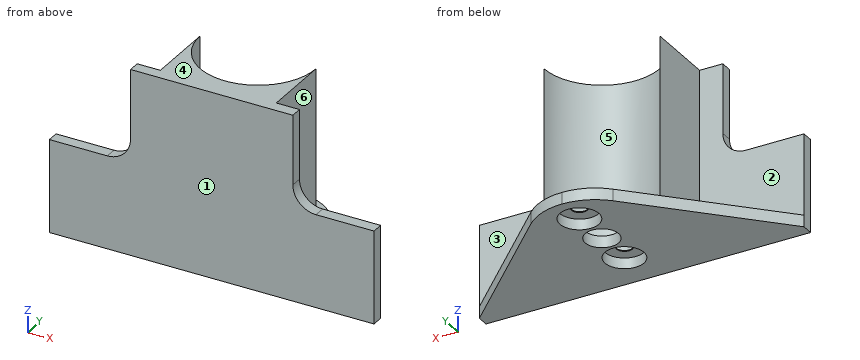
from build123d import *

# Parameters (mm, degrees)
BOSS_EXTRUDE1_DEPTH                              = 2.5
FILLET1_R                                        = 5
SKETCH3_W                                        = 70
SKETCH3_H                                        = 2.5
BOSS_EXTRUDE2_DEPTH                              = 30
CUT_EXTRUDE1_REACH                               = 62.725
BOSS_EXTRUDE3_DEPTH                              = 37.5
CUT_EXTRUDE3_REACH                               = 62.725
SKETCH10_R                                       = 3.6
CBORE_FOR_M3_HEX_HEAD_MACHINE_SCREW1_D           = 3.4
CBORE_FOR_M3_HEX_HEAD_MACHINE_SCREW1_CBORE_D     = 8.4
CBORE_FOR_M3_HEX_HEAD_MACHINE_SCREW1_CBORE_DEPTH = 2.3


with BuildPart() as part:
    # Sketch2 → Boss-Extrude1 (new body)
    with BuildSketch(Plane(origin=(0, 0, 0), x_dir=(1, 0, 0), z_dir=(0, 1, 0))):
        Polygon((-17.5, -30), (17.5, -30), (17.5, -10), (35, -10), (35, 10), (-35, 10), (-35, -10), (-17.5, -10), align=None)
    extrude(amount=BOSS_EXTRUDE1_DEPTH)

    # Fillet1
    fillet1_edges = [part.edges().sort_by_distance(p)[0] for p in [
        (-17.5, 1.25, 10),
        (17.5, 1.25, 10),
    ]]
    fillet(fillet1_edges, radius=FILLET1_R)

    # Sketch3 → Boss-Extrude2 (add)
    with BuildSketch(Plane(origin=(0, 2.5, 0), x_dir=(1, 0, 0), z_dir=(0, 1, 0))):
        with Locations((0, 8.75)):
            Rectangle(SKETCH3_W, SKETCH3_H)
    extrude(amount=BOSS_EXTRUDE2_DEPTH)

    # Sketch4 → Cut-Extrude1 (cut, up to next)
    with BuildSketch(Plane.XY.offset(-7.5), mode=Mode.PRIVATE) as cut_extrude1_sk1:
        with BuildLine():
            Line((-35, 32.5), (-35, 2.5))
            Line((-35, 2.5), (-8.868713205, 28.808854982))
            ThreePointArc((-8.868713205, 28.808854982), (-4.803088197, 31.54037884), (3.1e-08, 32.5))
            Line((3.1e-08, 32.5), (-35, 32.5))
        make_face()
    cut_extrude1_tool1 = extrude(cut_extrude1_sk1.sketch, amount=-CUT_EXTRUDE1_REACH, mode=Mode.PRIVATE) & part.part
    # Sketch4 → Cut-Extrude1 (cut, up to next)
    with BuildSketch(Plane.XY.offset(-7.5), mode=Mode.PRIVATE) as cut_extrude1_sk2:
        with BuildLine():
            Line((35, 32.5), (3.1e-08, 32.5))
            ThreePointArc((3.1e-08, 32.5), (4.803088226, 31.540378828), (8.868713205, 28.808854982))
            Line((8.868713205, 28.808854982), (35, 2.5))
            Line((35, 2.5), (35, 32.5))
        make_face()
    cut_extrude1_tool2 = extrude(cut_extrude1_sk2.sketch, amount=-CUT_EXTRUDE1_REACH, mode=Mode.PRIVATE) & part.part
    add(cut_extrude1_tool1.solids().sort_by_distance((-24.914818, 22.569917, -7.5))[0], mode=Mode.SUBTRACT)
    add(cut_extrude1_tool2.solids().sort_by_distance((24.914818, 22.569917, -7.5))[0], mode=Mode.SUBTRACT)

    # Sketch7 → Boss-Extrude3 (add)
    with BuildSketch(Plane.XY.offset(-7.5)):
        with BuildLine():
            Line((12.5, 17.5), (12.5, 2.5))
            Line((12.5, 2.5), (-12.5, 2.5))
            Line((-12.5, 2.5), (-12.5, 17.5))
            ThreePointArc((-12.5, 17.5), (0, 5), (12.5, 17.5))
        make_face()
    extrude(amount=BOSS_EXTRUDE3_DEPTH)

    # Sketch10 → Cut-Extrude3 (cut, up to next)
    with BuildSketch(Plane.XY.offset(-7.5), mode=Mode.PRIVATE) as cut_extrude3_sk1:
        with Locations((0, 17.5)):
            Circle(SKETCH10_R)
    cut_extrude3_tool1 = extrude(cut_extrude3_sk1.sketch, amount=-CUT_EXTRUDE3_REACH, mode=Mode.PRIVATE) & part.part
    add(cut_extrude3_tool1.solids().sort_by_distance((0, 17.5, -7.5))[0], mode=Mode.SUBTRACT)

    # CBORE for M3 Hex Head Machine Screw1 (through all)
    with Locations(Plane(origin=(0, 0, -10), x_dir=(-1, 0, 0), z_dir=(0, 0, -1))):
        with Locations((0, 26), (0, 9)):
            CounterBoreHole(CBORE_FOR_M3_HEX_HEAD_MACHINE_SCREW1_D / 2, CBORE_FOR_M3_HEX_HEAD_MACHINE_SCREW1_CBORE_D / 2, CBORE_FOR_M3_HEX_HEAD_MACHINE_SCREW1_CBORE_DEPTH)


solid = part.part
Can you work these out from the model? Positions are in its coordinate system, mm. Face numbers are marked on the shaded views. A direction names the side the tool comes from. Coordinates: 2 decimals unless noted, no trailing zeros. Loops run counter-clockwise (first coordinate to the right, second up) from the corner with the lowest first, then second, coordinate; pieces in that order, holes last. Notation, with made-up numbers: M -11.75,12.5 L 44.25,12.5 A14 cw 44.25,18.5 Z; hole C 84.5,46 d7. An arc over 180 degrees is marked long. Answer as CSV lines item,"result". Start each with the question number.
1. Suppose I cut it at B-B, the plane x = 1. List the corners of the cut face in (y, z) for me, plus the area to 3 significant figures.
2. Suppose I cut it at A-A, the plane y = 27. List the corners of the cut face in (x, z) for me, plus the area to 3 significant figures.
3. Suppose I cut it at C-C, the plane y = 11.5. List the corners of the cut face in (x, z) for me, plus the area to 3 significant figures.
4. For pin 1 Ø0.8 at (y, z) = (1.5, 25) entering from -X; pin 2 Ø6 at (y, z) = (12.5, 24) entering from +X; pin 3 Ø16.5 at (y, z) = (6.5, 18.5) entering from -X; pin 4 Ø6 at (x, y) = (0, 17.5) entering from -Z, each with a flat end and sliding along its axis, tell me the tip position at first contact or that it passes through.
5. Thinking about a two-plate mould opening in X: for the marked faces 4, 5 and 6, which applies, +X half, -X half, draft (parallel to the pull), parting line (faces both ways), or undercut?
6. If I drill on probe 1 along X at (y, z) = (9, -7); probe 2 along Y at (x, z) = (0, -7); probe 3 along Y at (x, z) = (16, -3), over which ranges is the centre line in solid material (lowest first)? Write a range as [from, to].
7. For the marked faces 1, 2 and 3, which set-ups out of +Z, -Z, +X, -X, +Y, -Y let a thin tool reach every point of the face, with its end or its side?
8. Suppose I cut it at D-D, the plane x = -30. List the corners of the cut face in (y, z) for me.
Output:
1,outline,"M 0,-10 L 4.92,-10 L 4.92,-7.7 L 7.63,-7.7 L 7.63,-7.5 L 5.04,-7.5 L 5.04,30 L 0,30 Z; M 10.37,-7.7 L 13.08,-7.7 L 13.08,-10 L 14.04,-10 L 14.04,-7.5 L 10.37,-7.5 Z; M 20.96,-10 L 21.92,-10 L 21.92,-7.7 L 24.63,-7.7 L 24.63,-7.5 L 20.96,-7.5 Z; M 27.37,-7.7 L 30.08,-7.7 L 30.08,-10 L 32.46,-10 L 32.46,-7.5 L 27.37,-7.5 Z"
1,area,"214 mm^2"
2,outline,"M -10.67,-10 L -4.08,-10 L -4.08,-7.7 L -1.37,-7.7 L -1.37,-7.5 L -10.67,-7.5 Z; M 1.37,-7.7 L 4.08,-7.7 L 4.08,-10 L 10.67,-10 L 10.67,-7.5 L 1.37,-7.5 Z"
2,area,"34.0 mm^2"
3,outline,"M -26.06,-10 L -3.37,-10 L -3.37,-7.7 L 3.37,-7.7 L 3.37,-10 L 26.06,-10 L 26.06,-7.5 L 12.5,-7.5 L 12.5,30 L 10.97,30 L 10.97,-7.5 L -10.97,-7.5 L -10.97,30 L -12.5,30 L -12.5,-7.5 L -26.06,-7.5 Z"
3,area,"230 mm^2"
4,pin 1,"stops at x = -17.5"
4,pin 2,"stops at x = 12.5"
4,pin 3,"stops at x = -19.15"
4,pin 4,"passes through"
5,face 4,"draft"
5,face 5,"undercut"
5,face 6,"+X half"
6,probe 1,"x = [-12.5, -9.17], [9.17, 12.5]"
6,probe 2,"y = [0, 5]"
6,probe 3,"y = [0, 2.5]"
7,face 1,"+Z, -Z, +X, -X, -Y"
7,face 2,"+Z, -X, +Y"
7,face 3,"+Z, +X, +Y"
8,outline,"M 0,-10 L 7.53,-10 L 7.53,-7.5 L 2.5,-7.5 L 2.5,10 L 0,10 Z"
